Here's the drawing with two shaded views (mm, measured from the low corner). I have some questions. Give positions to 0.01 mm unless a question says otherwise; leave off trailing zeros. Loops run counter-clockwise (first coordinate to the right, second up) from the corner with the lowest first, then second, coordinate; pieces in that order, holes last. Notation, with made-up numbers: (9, 5.5) -> (14, 5.5) arc R33 cw to (14, 40.5) -> close; hole circle Ø1 at (-11.5, 53). An arc over 180 degrees is marked (long way). Answer in a Markdown table with one row per item. Add a question column.
Item 1: If I drill on line 1 (Y direction, x = 8, z = 1.75); line 2 (X direction, y = 9.75, z = 2.75); line 3 (Y direction, x = 4.25, z = 2.75), over which ranges is the centre line in solid material (lowest first)?
Item 2: If we section it at D-D (x = 2.25): Write out the boundary of the cut face in (y, z).
Item 3: For P1, Ø2.5, axis at x = 8, y = 10.8, coming from the -Z side, with a flat end and sliding along its axis, tell me the tip position at first contact or that it passes through.
Item 4: We'd pull the mould along Y, two halves only. Please class the marked faces 1, 2 and 3: released by +Y, released by -Y, zero draft, split by the parting line, or undercut.
Item 5: If we section it at A-A (y = 9): Write out the boundary of the cut face in (x, z), then the cut area to 3 significant figures.
Item 6: If we section it at B-B (x = 8.25): Write out the boundary of the cut face in (y, z).
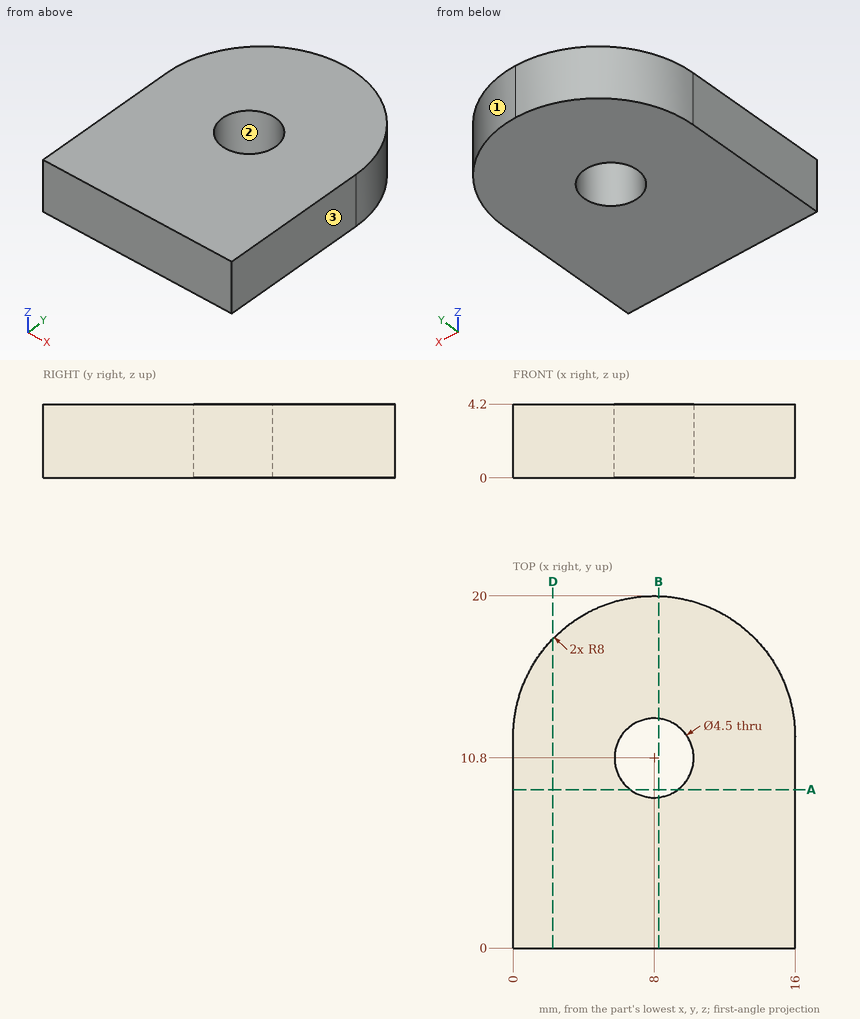
Recorded:
| question | item | result |
|---|---|---|
| 1 | line 1 | y = 0 to 8.55, 13.05 to 20 |
| 1 | line 2 | x = 0 to 6.01, 9.99 to 16 |
| 1 | line 3 | y = 0 to 19.07 |
| 2 | outline | (0, 0) -> (17.56, 0) -> (17.56, 4.2) -> (0, 4.2) -> close |
| 3 | P1 | passes through |
| 4 | face 1 | released by +Y |
| 4 | face 2 | undercut |
| 4 | face 3 | zero draft |
| 5 | outline | (0, 0) -> (6.65, 0) -> (6.65, 4.2) -> (0, 4.2) -> close; (9.35, 0) -> (16, 0) -> (16, 4.2) -> (9.35, 4.2) -> close |
| 5 | area | 55.9 mm^2 |
| 6 | outline | (0, 0) -> (8.56, 0) -> (8.56, 4.2) -> (0, 4.2) -> close; (13.04, 0) -> (20, 0) -> (20, 4.2) -> (13.04, 4.2) -> close |
